```python
from build123d import *

# Parameters (mm, degrees)
SKETCH_1_R      = 2
SKETCH_1_R_2    = 1
EXTRUDE_1_DEPTH = 100
SKETCH_2_W      = 0.5
SKETCH_2_H      = 3
SKETCH_4_W      = 0.5
SKETCH_4_H      = 50
SKETCH_5_W      = 0.5
SKETCH_5_H      = 4.2


with BuildPart() as part:
    # Эскиз1 → Бобышка-Вытянуть1 (new body)
    with BuildSketch(Plane(origin=(0, 0, 0), x_dir=(1, 0, 0), z_dir=(0, 1, 0))):
        Circle(SKETCH_1_R)
        Circle(SKETCH_1_R_2, mode=Mode.SUBTRACT)
    extrude(amount=EXTRUDE_1_DEPTH)

    # Эскиз2 → Вырез-Повернуть1 (revolve, cut)
    with BuildSketch(Plane.XY):
        with Locations((1.75, 1.5)):
            Rectangle(SKETCH_2_W, SKETCH_2_H)
        with Locations((1.75, 8.5)):
            Rectangle(SKETCH_2_W, SKETCH_2_H)
    revolve(axis=Axis((0, 0, 0), (0, 1, 0)), mode=Mode.SUBTRACT)

    # Эскиз4 → Вырез-Повернуть2 (revolve, cut)
    with BuildSketch(Plane.XY):
        with Locations((1.75, 75)):
            Rectangle(SKETCH_4_W, SKETCH_4_H)
    revolve(axis=Axis((0, 0, 0), (0, 1, 0)), mode=Mode.SUBTRACT)

    # Эскиз5 → Вырез-Повернуть3 (revolve, cut)
    with BuildSketch(Plane.XY):
        with Locations((1.75, 27.6)):
            Rectangle(SKETCH_5_W, SKETCH_5_H)
    revolve(axis=Axis((0, 0, 0), (0, 1, 0)), mode=Mode.SUBTRACT)


solid = part.part
```
The model under review builds one solid part; all positions refer to its coordinate system, in mm. A direction names the side the tool comes from. Round coordinates to 2 decimals unless told otherwise and drop trailing zeros. Order: outer loops, then holes, each group sorted by start corner. A loop starts at its lowest first (then second) coordinate and runs counter-clockwise, first axis right, second up.
(1) Mouldability with a two-part tool opening along Y and no side actions: class faces 4 (the face through (-1.5, 75.35, -0.07)), 5 (the face through (-1.5, 8.52, -0.07)) as released by +Y, released by -Y, zero draft, split by the parting line, or undercut.
Working result:
face 4: zero draft
face 5: undercut
(2) Wall thickness on L1, parallel to Y at x = 1.1, z = -1.55; L2, parallel to X at y = 71, z = 0: over which ranges is each line inside the solid? List them lowest first.
Working result:
L1: y = 3 to 7, 10 to 25.5, 29.7 to 50
L2: x = -1.5 to -1, 1 to 1.5
(3) For P1, Ø1.6, axis at x = 0, z = 0, coming from the +Y side (1 decimal); P2, Ø1.5, axis at y = 84, z = -0.5, coming from the -X side, all flat-tipped, find the tip position at first contact; note any pin that passes through.
Working result:
P1: passes through
P2: stops at x = -1.5
(4) Take a section at C-C, the plane y = 28. State the section outline as (x, z) points, plus the area to 3 significant figures.
Working result:
outline: circle Ø3 at (0, 0); hole circle Ø2 at (0, 0)
area: 3.93 mm2
(5) Tool access review of faces 1 (the face through (-1.5, 27.63, -0.07)), 2 (the face through (-1.5, 1.52, -0.07)), 3 (the face through (0, 49, 1)): name each direction out of +Z, -Z, +X, -X, +Y, -Y from which nothing blocks a thin tool from reaching the whole face with its end or side.
Working result:
face 1: none
face 2: -Y
face 3: +Y, -Y
